Design review of the part shown in the three views and the two pictorial views. Dimensions are in mm from the part's minimum x, y and z. A direction names the side the tool comes from. Coordinates: 2 decimals unless noted, no trailing zeros. Write each loop counter-clockwise with the first axis right and the second up, starting at its lowest first coordinate (ties: lowest second). Pieces come first, ordered by that corner, then holes. Notation, with made-up numbers: M 71,6 L 92,6 A13 ccw 92,20 Z; hole C 78.5,-16.75 d3. An arc over 180 degrees is marked long. One line per question, with ' | ' between items.
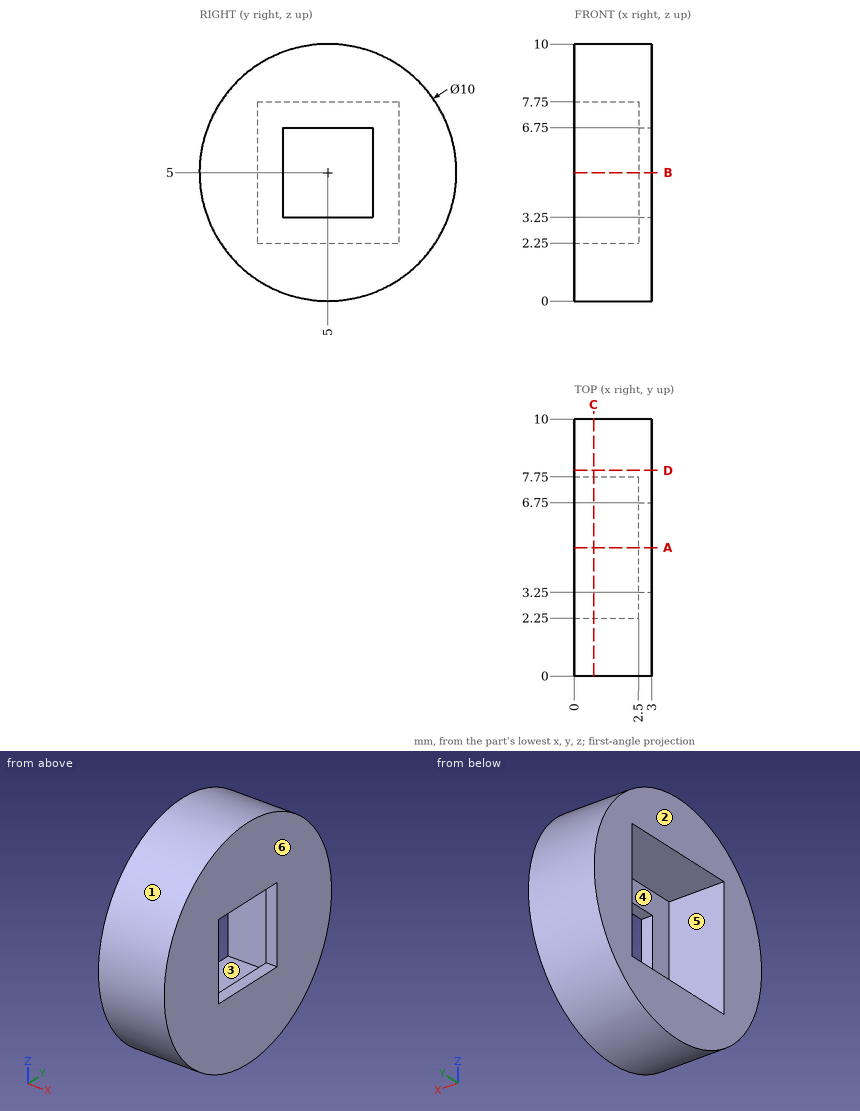
1. Take a section at A-A on y = 5. State the section outline as (x, z) points.
Computed values:
outline: M 0,0 L 3,0 L 3,3.25 L 2.5,3.25 L 2.5,2.25 L 0,2.25 Z; M 0,7.75 L 2.5,7.75 L 2.5,6.75 L 3,6.75 L 3,10 L 0,10 Z
2. For line 1 along X through (y, z) = (4.5, 2.5); line 2 along Z through (x, y) = (2.3, 2.75); line 3 along Z through (x, y) = (2.1, 6.5), list the stretches that pass through material, from the lowest coordinate up.
Computed values:
line 1: x = 2.5 to 3 | line 2: z = 0.53 to 2.25, 7.75 to 9.47 | line 3: z = 0.23 to 2.25, 7.75 to 9.77
3. Machinability: for the marked faces 5 and 6, which of the approach directions +Z, -Z, +X, -X, +Y, -Y give a long, thin tool a straight path to every point of the face, cutting with its end or side? Answer none if there is none.
Computed values:
face 5: -X | face 6: +Z, -Z, +X, +Y, -Y
4. Draft analysis for pull direction Y (two halves, no side actions). For the marked faces 1, 2, 3 and 4, state which applies: pulls with the +Y half, pulls with the -Y half, needs draft (parallel to the pull), parting line crosses it, or undercut.
Computed values:
face 1: parting line crosses it | face 2: needs draft | face 3: undercut | face 4: undercut
5. Take a section at D-D on y = 8. State the section outline as (x, z) points.
Computed values:
outline: M 0,1 L 3,1 L 3,9 L 0,9 Z
6. Clearance check with flat-ended pins moving along their axes: P1, Ø0.6, axis at x = 3, z = 5.5, coming from the -Y side; P2, Ø0.8, axis at x = 1, y = 6, coming from the +Z side. State where each tip first meets the part, or that it passes through.
Computed values:
P1: stops at y = 0 | P2: stops at z = 9.96
7. Take a section at C-C on x = 0.75. State the section outline as (y, z) points, plus the area to 3 significant figures.
Computed values:
outline: C 5,5 d10; hole M 2.25,2.25 L 7.75,2.25 L 7.75,7.75 L 2.25,7.75 Z | area: 48.3 mm2
